Build history of the part. All positions in model axes, mm. Face numbers are marked on the shaded views. Give positions to 0.01 mm unless a question says otherwise; leave off trailing zeros. Write each loop counter-clockwise with the first axis right and the second up, starting at its lowest first coordinate (ties: lowest second). Pieces come first, ordered by that corner, then holes. Notation, with made-up numbers: (83.25, 77) -> (128.25, 77) arc R16 ccw to (128.25, 90) -> close; hole circle Ø11 at (-20.75, -29). An arc over 180 degrees is marked (long way). One line per question, with ' | ' between items. Start each with the question number.
(1) Band-saw the part on D-D, the plane z = -15. Give the cut face in (x, y).
(2) Drill centre lines: probe 1 along X at (y, z) = (2.9, -30.8) (3 decimals); probe 2 along X at (y, z) = (4, -44.45); probe 3 along Z at (x, y) = (20, 2.85). Where is each one in solid material? Low to high. Write a range as from..to.
(3) Pin check, flat tips, straight feed: P1, Ø1.5, axis at x = 15.875, z = -30.8, coming from the +Y side; P2, Ø1.5, axis at x = 65.5, y = 1, coming from the -Z side. Stop position of each tip, or through.
(4) Band-saw the part on A-A, the plane x = 38.1. Give the cut face in (y, z), and give its area (3 significant figures).
(5) Pull direction Z, two halves, no side cores. Call the marked faces 1, 2 and 3: released by +Z, released by -Z, zero draft, split by the parting line, or undercut.
(6) Band-saw the part on C-C, the plane y = 4.4. Count the separate pieces of the cut face and the enclosed holes in it, and give its area (3 significant figures).
(7) Band-saw the part on B-B, the plane z = -31. Give the cut face in (x, y).
from build123d import *

# Parameters (mm, degrees)
SKETCH1_R           = 8
BOSS_EXTRUDE1_DEPTH = 5.8
SKETCH2_R           = 1.3
CUT_EXTRUDE1_DEPTH  = 92.764481146
SKETCH14_R          = 1.25
M3_TAP_DEPTH        = 92.764481146
SKETCH15_R          = 2.65
M5_THROUGH_DEPTH    = 92.764481146
CUT_EXTRUDE2_DEPTH  = 92.764481146
FILLET2_R           = 6.35
SKETCH13_R          = 1.5
CUT_EXTRUDE3_DEPTH  = 92.764481146
MOVE_FACE1_BY       = 0.08
MOVE_FACE1_2_BY     = 0.08
MOVE_FACE1_3_BY     = 0.08
MOVE_FACE1_4_BY     = 0.08
MOVE_FACE1_5_BY     = 0.08
MOVE_FACE1_6_BY     = 0.08
MOVE_FACE1_7_BY     = 0.08
MOVE_FACE1_8_BY     = 0.08
MOVE_FACE1_9_BY     = 0.08
MOVE_FACE1_10_BY    = 0.08
MOVE_FACE1_11_BY    = 0.08
MOVE_FACE1_12_BY    = 0.08
MOVE_FACE1_13_BY    = 0.08
MOVE_FACE1_14_BY    = 0.08
MOVE_FACE1_15_BY    = 0.08
MOVE_FACE1_16_BY    = 0.08


with BuildPart() as part:
    # Sketch1 → Boss-Extrude1 (new body)
    with BuildSketch(Plane(origin=(0, 0, 0), x_dir=(1, 0, 0), z_dir=(0, 1, 0))):
        Polygon((0, 0), (76.2, 0), (76.2, 50.8), (38.1, 50.8), (0, 50.8), align=None)
        with Locations(Location((38.1, 30.8, 0), (0, 0, 270))):
            Circle(SKETCH1_R, mode=Mode.SUBTRACT)
    extrude(amount=BOSS_EXTRUDE1_DEPTH)

    # Sketch2 → Cut-Extrude1 (cut, through all)
    with BuildSketch(Plane(origin=(0, 5.8, 0), x_dir=(1, 0, 0), z_dir=(0, 1, 0))):
        with Locations(Location((15.875, 30.8, 0), (0, 0, 270))):
            Circle(SKETCH2_R)
        with Locations(Location((60.325, 30.8, 0), (0, 0, 270))):
            Circle(SKETCH2_R)
    extrude(amount=-CUT_EXTRUDE1_DEPTH, mode=Mode.SUBTRACT)

    # Sketch14 → M3-tap (cut, through all)
    with BuildSketch(Plane.XZ):
        with Locations(Location((57.15, -44.45, 0), (0, 0, 270))):
            Circle(SKETCH14_R)
        with Locations(Location((19.05, -44.45, 0), (0, 0, 270))):
            Circle(SKETCH14_R)
        with Locations(Location((19.05, -17.15, 0), (0, 0, 270))):
            Circle(SKETCH14_R)
        with Locations(Location((57.15, -17.15, 0), (0, 0, 270))):
            Circle(SKETCH14_R)
    extrude(amount=-M3_TAP_DEPTH, mode=Mode.SUBTRACT)

    # Sketch15 → M5-through (cut, through all)
    with BuildSketch(Plane.XZ):
        with Locations(Location((69.85, -24.45004, 0), (0, 0, 270))):
            Circle(SKETCH15_R)
        with Locations(Location((69.85, -6.35, 0), (0, 0, 270))):
            Circle(SKETCH15_R)
        with Locations(Location((48.683333333, -6.35, 0), (0, 0, 270))):
            Circle(SKETCH15_R)
        with Locations(Location((27.516666667, -6.35, 0), (0, 0, 270))):
            Circle(SKETCH15_R)
        with Locations(Location((6.35, -6.35, 0), (0, 0, 270))):
            Circle(SKETCH15_R)
        with Locations(Location((6.35, -24.45004, 0), (0, 0, 270))):
            Circle(SKETCH15_R)
    extrude(amount=-M5_THROUGH_DEPTH, mode=Mode.SUBTRACT)

    # Sketch12 → Cut-Extrude2 (cut, through all)
    with BuildSketch(Plane(origin=(0, 5.8, 0), x_dir=(1, 0, 0), z_dir=(0, 1, 0))):
        Polygon((0, 50.8), (12.7, 50.8), (12.7, 37.15), (0, 24.45), align=None)
        Polygon((63.5, 50.8), (63.5, 37.15), (76.2, 24.45), (76.2, 50.8), align=None)
    extrude(amount=-CUT_EXTRUDE2_DEPTH, mode=Mode.SUBTRACT)

    # Fillet2
    fillet2_edges = [part.edges().sort_by_distance(p)[0] for p in [
        (0, 2.9, -24.45),
        (12.7, 2.9, -50.8),
        (12.7, 2.9, -37.15),
        (76.2, 2.9, 0),
        (63.5, 2.9, -50.8),
        (0, 2.9, 0),
        (76.2, 2.9, -24.45),
        (63.5, 2.9, -37.15),
    ]]
    fillet(fillet2_edges, radius=FILLET2_R)

    # Sketch13 → Cut-Extrude3 (cut, through all)
    with BuildSketch(Plane.XZ):
        with Locations(Location((69.85, -15.40002, 0), (0, 0, 270))):
            Circle(SKETCH13_R)
        with Locations(Location((38.1, -6.35, 0), (0, 0, 270))):
            Circle(SKETCH13_R)
        with Locations(Location((6.35, -15.40002, 0), (0, 0, 270))):
            Circle(SKETCH13_R)
    extrude(amount=-CUT_EXTRUDE3_DEPTH, mode=Mode.SUBTRACT)

    # Move Face1: a curved face moved outward by 0.08
    add(Solid.thicken(part.faces().sort_by_distance((38.1, 2.9, -38.8))[0], MOVE_FACE1_BY))

    # Move Face1 2: a curved face moved outward by 0.08
    add(Solid.thicken(part.faces().sort_by_distance((15.875, 2.9, -32.1))[0], MOVE_FACE1_2_BY))

    # Move Face1 3: a curved face moved outward by 0.08
    add(Solid.thicken(part.faces().sort_by_distance((60.325, 2.9, -32.1))[0], MOVE_FACE1_3_BY))

    # Move Face1 4: a curved face moved outward by 0.08
    add(Solid.thicken(part.faces().sort_by_distance((57.15, 2.9, -43.2))[0], MOVE_FACE1_4_BY))

    # Move Face1 5: a curved face moved outward by 0.08
    add(Solid.thicken(part.faces().sort_by_distance((19.05, 2.9, -43.2))[0], MOVE_FACE1_5_BY))

    # Move Face1 6: a curved face moved outward by 0.08
    add(Solid.thicken(part.faces().sort_by_distance((19.05, 2.9, -15.9))[0], MOVE_FACE1_6_BY))

    # Move Face1 7: a curved face moved outward by 0.08
    add(Solid.thicken(part.faces().sort_by_distance((57.15, 2.9, -15.9))[0], MOVE_FACE1_7_BY))

    # Move Face1 8: a curved face moved outward by 0.08
    add(Solid.thicken(part.faces().sort_by_distance((69.85, 2.9, -21.80004))[0], MOVE_FACE1_8_BY))

    # Move Face1 9: a curved face moved outward by 0.08
    add(Solid.thicken(part.faces().sort_by_distance((69.85, 2.9, -3.7))[0], MOVE_FACE1_9_BY))

    # Move Face1 10: a curved face moved outward by 0.08
    add(Solid.thicken(part.faces().sort_by_distance((48.683333333, 2.9, -3.7))[0], MOVE_FACE1_10_BY))

    # Move Face1 11: a curved face moved outward by 0.08
    add(Solid.thicken(part.faces().sort_by_distance((27.516666667, 2.9, -3.7))[0], MOVE_FACE1_11_BY))

    # Move Face1 12: a curved face moved outward by 0.08
    add(Solid.thicken(part.faces().sort_by_distance((6.35, 2.9, -3.7))[0], MOVE_FACE1_12_BY))

    # Move Face1 13: a curved face moved outward by 0.08
    add(Solid.thicken(part.faces().sort_by_distance((6.35, 2.9, -21.80004))[0], MOVE_FACE1_13_BY))

    # Move Face1 14: a curved face moved outward by 0.08
    add(Solid.thicken(part.faces().sort_by_distance((69.85, 2.9, -13.90002))[0], MOVE_FACE1_14_BY))

    # Move Face1 15: a curved face moved outward by 0.08
    add(Solid.thicken(part.faces().sort_by_distance((38.1, 2.9, -4.85))[0], MOVE_FACE1_15_BY))

    # Move Face1 16: a curved face moved outward by 0.08
    add(Solid.thicken(part.faces().sort_by_distance((6.35, 2.9, -13.90002))[0], MOVE_FACE1_16_BY))


solid = part.part
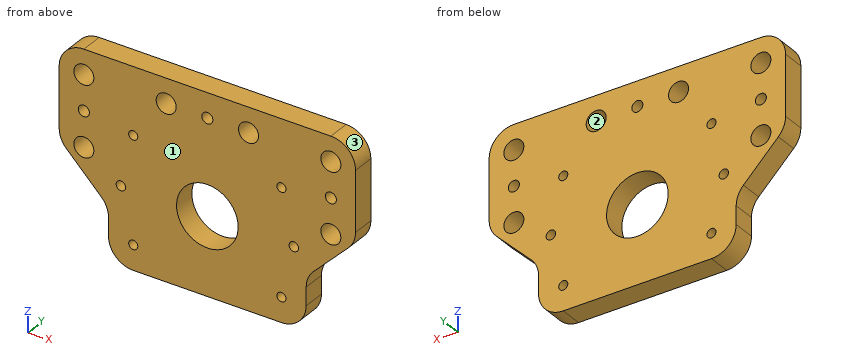
Results:
1) outline: (0, 0) -> (4.99, 0) -> (4.99, 5.8) -> (0, 5.8) -> close; (7.71, 0) -> (68.49, 0) -> (68.49, 5.8) -> (7.71, 5.8) -> close; (71.21, 0) -> (76.2, 0) -> (76.2, 5.8) -> (71.21, 5.8) -> close
2) probe 1: x = 6.35..14.655, 17.095..30.18, 46.02..59.105, 61.545..69.85 | probe 2: x = 12.7..17.88, 20.22..55.98, 58.32..63.5 | probe 3: z = -50.8..-45.13, -43.77..-17.83, -16.47..0
3) P1: passes through | P2: stops at z = -36
4) outline: (0, -50.8) -> (5.8, -50.8) -> (5.8, -38.72) -> (0, -38.72) -> close; (0, -22.88) -> (5.8, -22.88) -> (5.8, -7.77) -> (0, -7.77) -> close; (0, -4.93) -> (5.8, -4.93) -> (5.8, 0) -> (0, 0) -> close | area: 186 mm²
5) face 1: zero draft | face 2: undercut | face 3: released by +Z
6) separate pieces: 1 | enclosed holes: 16 | area: 2,960 mm²
7) outline: (6.55, 0) -> (14.67, 0) -> (14.67, 5.8) -> (6.55, 5.8) -> close; (17.08, 0) -> (30.18, 0) -> (30.18, 5.8) -> (17.08, 5.8) -> close; (46.02, 0) -> (59.12, 0) -> (59.12, 5.8) -> (46.02, 5.8) -> close; (61.53, 0) -> (69.65, 0) -> (69.65, 5.8) -> (61.53, 5.8) -> close
